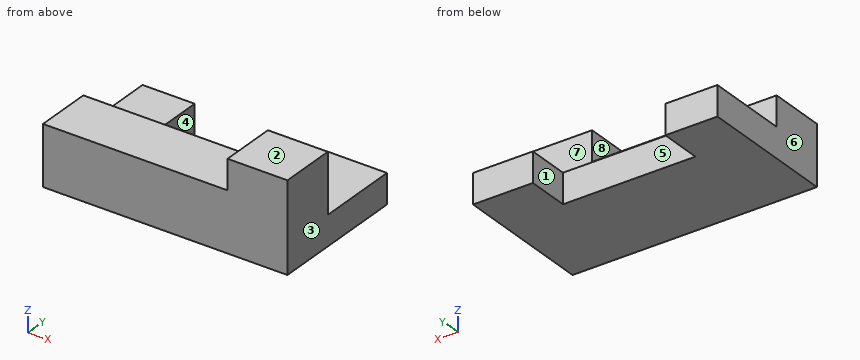
```python
from build123d import *

# Parameters (mm, degrees)
EXTRUDE_1_DEPTH = 10
SKETCH_1_3_W    = 20.109572138
SKETCH_1_3_H    = 18.992234217
EXTRUDE_2_DEPTH = 30
SKETCH_1_4_W    = 61.971467386
SKETCH_1_4_H    = 18.992234217
EXTRUDE_3_DEPTH = 20


with BuildPart() as part:
    # Sketch 1 → Extrude 1 (new body)
    with BuildSketch(Plane.XY):
        Polygon((-21.993563511, 13.719879355), (-21.993563511, 27.903717876), (-39.506294724, 27.903717876), (-39.506294724, 0), (42.5747448, 0), (42.5747448, 27.903717876), (22.465172662, 27.903717876), (22.465172662, 13.719879355), align=None)
    extrude(amount=EXTRUDE_1_DEPTH)

    # Sketch 1_3 → Extrude 2 (add)
    with BuildSketch(Plane.XY):
        with Locations((32.519958731, -9.496117109)):
            Rectangle(SKETCH_1_3_W, SKETCH_1_3_H)
    extrude(amount=EXTRUDE_2_DEPTH)

    # Sketch 1_4 → Extrude 3 (add)
    with BuildSketch(Plane.XY):
        with Locations((-8.520561031, -9.496117109)):
            Rectangle(SKETCH_1_4_W, SKETCH_1_4_H)
    extrude(amount=EXTRUDE_3_DEPTH)


solid = part.part
```
Input: part model. Units: mm. Frame: model coordinates. Face numbers are marked on the shaded views. A direction names the side the tool comes from. Round coordinates to 2 decimals unless told otherwise and drop trailing zeros. Order: outer loops, then holes, each group sorted by start corner. A loop starts at its lowest first (then second) coordinate and runs counter-clockwise, first axis right, second up. Notation, with made-up numbers: (10.25, -26.75) - (45.25, -26.75) arc R30 cw to (45.25, -2.75) - close; hole circle Ø5 at (70.5, -17). An arc over 180 degrees is marked (long way). Answer in a Markdown table with one row per item.
Item 1: Section query C-C (x = 31). Return the cut outline in (y, z), then the cut area to 3 significant figures.
Model answer:
| item | result |
|---|---|
| outline | (-18.99, 0) - (27.9, 0) - (27.9, 10) - (0, 10) - (0, 30) - (-18.99, 30) - close |
| area | 849 mm² |
Item 2: Mould query, pull axis X, two halves, no side actions, for the marked faces 1, 2, 3 and 4. Classes: released by +X, released by -X, zero draft, split by the parting line, or undercut.
Model answer:
| item | result |
|---|---|
| face 1 | undercut |
| face 2 | zero draft |
| face 3 | released by +X |
| face 4 | undercut |
Item 3: Section query D-D (y = -6). Return the cut outline in (x, z).
Model answer:
| item | result |
|---|---|
| outline | (-39.51, 0) - (42.57, 0) - (42.57, 30) - (22.47, 30) - (22.47, 20) - (-39.51, 20) - close |
Item 4: Reachability of the marked faces 5, 6, 7 and 8 from +Z, -Z, +X, -X, +Y, -Y: full face, straight path, thin tool, end or side. Return the list, or none.
Model answer:
| item | result |
|---|---|
| face 5 | +Z, -Z, +Y |
| face 6 | +Z, -Z, -X, +Y, -Y |
| face 7 | +Z, +X, -X, +Y |
| face 8 | +Z, -X, +Y, -Y |
Item 5: Line query: line 1 (X direction, y = 18.5, z = 2); line 2 (Z direction, x = -23.5, y = 17.5); line 3 (Y direction, x = 22, z = 14.75). Output: solid intervals per line, ascending.
Model answer:
| item | result |
|---|---|
| line 1 | x = -39.51 to -21.99, 22.47 to 42.57 |
| line 2 | z = 0 to 10 |
| line 3 | y = -18.99 to 0 |
Item 6: Pin query (flat end, axial travel): pin 1 (3 mm diameter, centred on x = -1, z = 7, fed in from +Y); pin 2 (9.5 mm diameter, centred on x = -17.5, y = -5.5, fed in from +Z); pin 3 (14 mm diameter, centred on x = 18.5, y = 20.5, fed in from +Z); pin 4 (3 mm diameter, centred on y = 18.5, z = 12, fed in from -X). Return the tip coordinate at first contact, or that it passes through.
Model answer:
| item | result |
|---|---|
| pin 1 | stops at y = 13.72 |
| pin 2 | stops at z = 20 |
| pin 3 | stops at z = 10 |
| pin 4 | passes through |
Item 7: Section query B-B (z = 2.75). Return the cut outline in (x, y).
Model answer:
| item | result |
|---|---|
| outline | (-39.51, -18.99) - (42.57, -18.99) - (42.57, 27.9) - (22.47, 27.9) - (22.47, 13.72) - (-21.99, 13.72) - (-21.99, 27.9) - (-39.51, 27.9) - close |
Item 8: Section query A-A (y = 22). Return the cut outline in (x, z), then the cut area to 3 significant figures.
Model answer:
| item | result |
|---|---|
| outline | (-39.51, 0) - (-21.99, 0) - (-21.99, 10) - (-39.51, 10) - close; (22.47, 0) - (42.57, 0) - (42.57, 10) - (22.47, 10) - close |
| area | 376 mm² |
